Check sheet for the modelled part. Datum: model origin and axes. Units: mm. Face numbers are marked on the shaded views. Round coordinates to 2 decimals unless told otherwise and drop trailing zeros. Loops run counter-clockwise (first coordinate to the right, second up) from the corner with the lowest first, then second, coordinate; pieces in that order, holes last. Notation, with made-up numbers: (49.25, -21.75) - (97.25, -21.75) arc R36 ccw to (97.25, 14.25) - close; hole circle Ø1 at (43.25, -29). An arc over 180 degrees is marked (long way). Answer in a Markdown table with one row per item. Add a question column.
(1) Cross-section at B-B on x = 0. Enter the section's corners in (y, z), then the cut area to 3 significant figures.
(2) Gauge pin test, flat ends, axial feed: pin 1 (2 mm diameter, centred on x = 12.5, z = -6.5, fed in from +Y); pin 2 (4 mm diameter, centred on y = 10, z = -19.5, fed in from +X); pin 3 (6 mm diameter, centred on x = 3, z = -8.5, fed in from +Y); pin 4 (10 mm diameter, centred on x = 18, z = 7.5, fed in from -Y). Record the tip position at first contact, or that the pin passes through.
(3) Cross-section at A-A on z = 0. Enter the section's corners in (x, y), then the cut area to 3 significant figures.
(4) Mould release check, pull along X, two halves, no side actions. Record for the marked faces 1 and 2: +X half, -X half, draft (parallel to the pull), parting line (faces both ways), or undercut.
(5) Cross-section at C-C on y = 13.5. Enter the section's corners in (x, z), then the cut area to 3 significant figures.
(6) Thickness scan on line 1 along X through (y, z) = (20.5, 0); line 2 along X through (y, z) = (22.5, -21); line 3 along Z through (x, y) = (14, 27). Record the ranges inside material, lowest first.
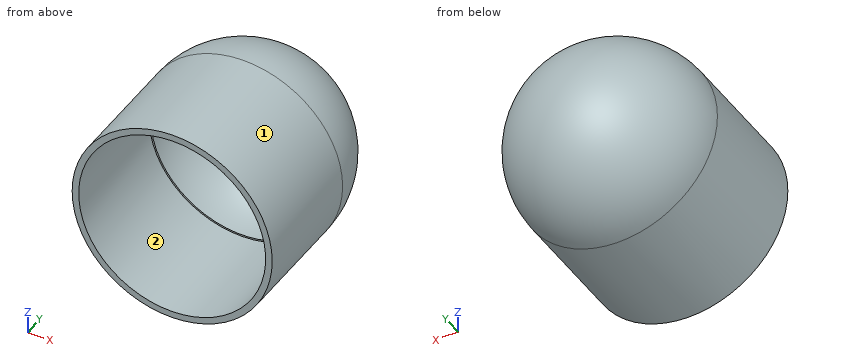
from build123d import *

# Parameters (mm, degrees)
SKETCH2_R           = 24.5
BOSS_EXTRUDE1_DEPTH = 30
REVOLVE_THIN1_ANGLE = 180
SKETCH6_R           = 22.9
CUT_EXTRUDE1_DEPTH  = 30


with BuildPart() as part:
    # Sketch2 → Boss-Extrude1 (new body)
    with BuildSketch(Plane(origin=(0, 0, 0), x_dir=(1, 0, 0), z_dir=(0, 1, 0))):
        with Locations(Location((0, 0, 0), (0, 0, 270))):
            Circle(SKETCH2_R)
    extrude(amount=BOSS_EXTRUDE1_DEPTH)

    # Sketch4 → Revolve-Thin1 (revolve)
    with BuildSketch(Plane(origin=(0, 30, 0), x_dir=(1, 0, 0), z_dir=(0, 1, 0))):
        with BuildLine():
            ThreePointArc((24.5, 0), (0, -24.5), (-24.5, 0))
            Line((-24.5, 0), (-22.5, 0))
            ThreePointArc((-22.5, 0), (0, -22.5), (22.5, 0))
            Line((22.5, 0), (24.5, 0))
        make_face()
    revolve(axis=Axis((0, 30, 0), (-1, 0, 0)), revolution_arc=REVOLVE_THIN1_ANGLE)

    # Sketch6 → Cut-Extrude1 (cut)
    with BuildSketch(Plane.XZ):
        with Locations(Location((0, 0, 0), (0, 0, 270))):
            Circle(SKETCH6_R)
    extrude(amount=-CUT_EXTRUDE1_DEPTH, mode=Mode.SUBTRACT)


solid = part.part
Answers:
| question | item | result |
|---|---|---|
| 1 | outline | (0, -24.5) - (30, -24.5) arc R24.5 ccw to (30, 24.5) - (0, 24.5) - (0, 22.9) - (30, 22.9) - (30, 22.5) arc R22.5 cw to (30, -22.5) - (30, -22.9) - (0, -22.9) - close |
| 1 | area | 244 mm^2 |
| 2 | pin 1 | stops at y = 50.71 |
| 2 | pin 2 | stops at x = 17.15 |
| 2 | pin 3 | stops at y = 53.75 |
| 2 | pin 4 | stops at y = 0 |
| 3 | outline | (-24.5, 0) - (-22.9, 0) - (-22.9, 30) - (-22.5, 30) arc R22.5 cw to (22.5, 30) - (22.9, 30) - (22.9, 0) - (24.5, 0) - (24.5, 30) arc R24.5 ccw to (-24.5, 30) - close |
| 3 | area | 244 mm^2 |
| 4 | face 1 | parting line |
| 4 | face 2 | undercut |
| 5 | outline | circle Ø49 at (0, 0); hole circle Ø45.8 at (0, 0) |
| 5 | area | 238 mm^2 |
| 6 | line 1 | x = -24.5 to -22.9, 22.9 to 24.5 |
| 6 | line 2 | x = -12.62 to -9.13, 9.13 to 12.62 |
| 6 | line 3 | z = -20.11 to -18.12, 18.12 to 20.11 |
